```python
from build123d import *

# Parameters (mm, degrees)
SKETCH1_R          = 9.525
EXTRUDE1_DEPTH     = 7.9375
CUT_EXTRUDE1_DEPTH = 3.96875
SKETCH18_R         = 3.666174209
CUT_EXTRUDE4_DEPTH = 1.322916667
CUT_EXTRUDE4_DRAFT = -45
SKETCH4_R          = 6.35
EXTRUDE2_DEPTH     = 63.5
SKETCH5_R          = 4.7625
EXTRUDE3_DEPTH     = 15.875
CHAMFER1_SIZE      = 1.5875
CHAMFER2_SIZE      = 0.529166667
CHAMFER3_SIZE      = 0.396875


with BuildPart() as part:
    # Sketch1 → Extrude1 (new body)
    with BuildSketch(Plane(origin=(0, 0, 0), x_dir=(1, 0, 0), z_dir=(0, 1, 0))):
        with Locations(Location((0, 0, 0), (0, 0, 270))):
            Circle(SKETCH1_R)
    extrude(amount=EXTRUDE1_DEPTH)

    # Sketch2 → Cut-Extrude1 (cut)
    with BuildSketch(Plane(origin=(0, 7.9375, 0), x_dir=(-1, 0, 0), z_dir=(0, 1, 0))):
        Polygon((0, -3.666174209), (3.175, -1.833087105), (3.175, 1.833087105), (0, 3.666174209), (-3.175, 1.833087105), (-3.175, -1.833087105), align=None)
    extrude(amount=-CUT_EXTRUDE1_DEPTH, mode=Mode.SUBTRACT)


with BuildPart() as cut_extrude4_tool:
    # Sketch18 → Cut-Extrude4 (with draft: the straight prism first)
    with BuildSketch(Plane(origin=(0, 7.9375, 0), x_dir=(1, 0, 0), z_dir=(0, 1, 0))):
        Circle(SKETCH18_R)
    extrude(amount=-CUT_EXTRUDE4_DEPTH)
    # Cut-Extrude4: the draft: its side faces are tilted about the plane it starts from
    cut_extrude4_sides = [cut_extrude4_tool.faces().sort_by_distance(p)[0] for p in [
        (-3.666174209, 7.276041667, 0),
    ]]
    draft(cut_extrude4_sides, Plane(origin=(0, 7.9375, 0), x_dir=(1, 0, 0), z_dir=(0, 1, 0)), CUT_EXTRUDE4_DRAFT)


with BuildPart() as part_1:
    add(part.part)

    # Cut-Extrude4: cut by cut_extrude4_tool
    add(cut_extrude4_tool.part, mode=Mode.SUBTRACT)

    # Sketch4 → Extrude2 (add)
    with BuildSketch(Plane.XZ.offset(63.5)):
        with Locations(Location((0, 0, 0), (0, 0, 270))):
            Circle(SKETCH4_R)
    extrude(amount=-EXTRUDE2_DEPTH)

    # Sketch5 → Extrude3 (add)
    with BuildSketch(Plane.XZ.offset(63.5)):
        with Locations(Location((0, 0, 0), (0, 0, 270))):
            Circle(SKETCH5_R)
    extrude(amount=EXTRUDE3_DEPTH)

    # Chamfer1
    chamfer1_edges = [part_1.edges().sort_by_distance(p)[0] for p in [
        (0, -79.375, 4.7625),
    ]]
    chamfer(chamfer1_edges, length=CHAMFER1_SIZE)

    # Sketch17 → Cut-Revolve1 (revolve, cut)
    with BuildSketch(Plane.XY):
        with BuildLine():
            Line((4.862800608, -63.5), (6.35, -63.5))
            Line((6.35, -63.5), (6.35, -67.46875))
            Line((6.35, -67.46875), (6.35, -70.146574392))
            Line((6.35, -70.146574392), (3.672175608, -67.46875))
            Line((3.672175608, -67.46875), (3.672175608, -64.690625))
            ThreePointArc((3.672175608, -64.690625), (4.020901597, -63.848725989), (4.862800608, -63.5))
        make_face()
    revolve(axis=Axis((0, 0, 0), (0, -1, 0)), mode=Mode.SUBTRACT)

    # Chamfer2
    chamfer2_edges = [part_1.edges().sort_by_distance(p)[0] for p in [
        (0, -63.5, 6.35),
    ]]
    chamfer(chamfer2_edges, length=CHAMFER2_SIZE)

    # Chamfer3
    chamfer3_edges = [part_1.edges().sort_by_distance(p)[0] for p in [
        (0, 7.9375, -9.525),
    ]]
    chamfer(chamfer3_edges, length=CHAMFER3_SIZE)


solid = part_1.part
```
The model under review builds one solid part; all positions refer to its coordinate system, in mm. A direction names the side the tool comes from. Round coordinates to 2 decimals unless told otherwise and drop trailing zeros. Write each loop counter-clockwise with the first axis right and the second up, starting at its lowest first coordinate (ties: lowest second). Pieces come first, ordered by that corner, then holes.
(1) Insertion check: pin 1 (9.5 mm diameter, centred on x = 4, z = 1, fed in from -Y) (3 decimals); pin 2 (1 mm diameter, centred on y = -61.5, z = -2.5, fed in from -X); pin 3 (6 mm diameter, centred on y = -30.5, z = -3, fed in from +X); pin 4 (3 mm diameter, centred on y = -46, z = 3, fed in from -X). Each pin has a flat end and moves straight along its axis. Give the tip position at first contact, or say it passes through.
(2) Wall thickness on L1, parallel to Y at x = 5, z = 7; L2, parallel to Y at x = 1.5, z = -2.25 (3 decimals); L3, parallel to Z at x = -5.5, y = -59: over which ranges is each line inside the solid? List them lowest first.
(3) We need section C-C on y = -18.5. Give the boundary of the cut face in (x, z).
(4) We need section B-B on y = -71. Give the boundary of the cut face in (x, z) (1 decimal).
(5) Machinability: for faces 1 (the cylindrical face through (-5.796, 3.718, -7.559)), 2 (the flat face through (-1.61, 5.981, 2.737)), 3 (the flat face through (0, -63.5, 5)), which of the approach directions +Z, -Z, +X, -X, +Y, -Y give a long, thin tool a straight path to every point of the face, cutting with its end or side? Answer none if there is none.
(6) Mouldability with a two-part tool opening along Y and no side actions: class faces 4 (the cylindrical face through (-0.796, -66.06, -3.585)), 5 (the flat face through (-1.57, 5.98, -2.76)), 6 (the conical face through (-1.734, 7.695, 2.953)) as +Y half, -Y half, draft (parallel to the pull), parting line (faces both ways), or undercut.
Findings below:
1. pin 1: stops at y = -79.375
1. pin 2: stops at x = -6.03
1. pin 3: stops at x = 6.35
1. pin 4: stops at x = -6.17
2. L1: y = 0 to 7.94
2. L2: y = -79.375 to 3.969
2. L3: z = -3.17 to 3.17
3. outline: circle Ø12.7 at (0, 0)
4. outline: circle Ø9.5 at (0, 0)
5. face 1: +Y, -Y
5. face 2: +Y
5. face 3: -Y
6. face 4: undercut
6. face 5: draft
6. face 6: +Y half
